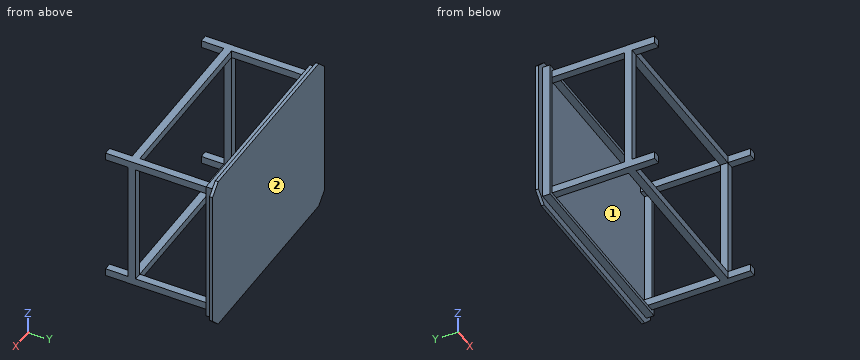
Autodesk Inventor part; units mm, degrees
ref_plane "Plano de trabajo2" through (-617.5, -580, 460) normal (0, 1, 0) x (1, 0, 0)
ref_plane "YZ Plane" through (0, 0, 0) normal (1, 0, 0) x (0, 1, 0)
ref_plane "XZ Plane" through (0, 0, 0) normal (0, 1, 0) x (-1, 0, 0)
sketch "Boceto1" plane through (0, 0, 0) normal (0, 1, 0) x (-1, 0, 0)
  line L0 (692.5, 535) -> (-692.5, 535)
  line L1 (-692.5, 535) -> (-692.5, -535)
  line L2 (-692.5, -535) -> (692.5, -535)
  line L3 (692.5, -535) -> (692.5, 535)
  line L4 (622.5, 535) -> (692.5, 465)
  line L5 (692.5, 0) -> (-692.5, 0)
  line L6 (0, 535) -> (0, -535)
  line L7 (622.5, -535) -> (692.5, -465)
  line L8 (-622.5, 535) -> (-692.5, 465)
  line L9 (-622.5, -535) -> (-692.5, -465)
  arc A0 (-507.7191, -338.4764) -> (-457.7841, -385.927) centre (-457.7841, -335.927) ccw
  line L10 (-457.7841, -385.927) -> (492.0857, -385.927)
  arc A1 (492.0857, -385.927) -> (542.0206, -333.3776) centre (492.0857, -335.927) ccw
  line L11 (542.0206, -333.3776) -> (507.8137, 336.6224)
  arc A2 (507.8137, 336.6224) -> (457.8787, 384.073) centre (457.8787, 334.073) ccw
  line L12 (457.8787, 384.073) -> (-491.991, 384.073)
  arc A3 (-491.991, 384.073) -> (-541.926, 331.5236) centre (-491.991, 334.073) ccw
  line L13 (-541.926, 331.5236) -> (-507.7191, -338.4764)
  point P0 (0, 0)
  point P1 (-692.5, -465)
  point P2 (622.5, -535)
  point P3 (692.5, -465)
  dimension "d0" = 1070
  dimension "d1" = 1385
  dimension "d2" = 692.5
  dimension "d3" = 535
  dimension "d4" = 70
  dimension "d5" = 70
  dimension "d27" = 770
extrude "Extrusión1" add sketch "Boceto1" along normal blind 20 contours L4 L3 L5 L11 A2 L12 L6 L0 | L6 L12 A3 L13 L5 L1 L8 L0 | L3 L7 L2 L6 L10 A1 L11 L5 | L12 A2 L11 L5 L6 | L6 L5 L13 A3 L12 | L11 A1 L10 L6 L5 | L6 L10 A0 L13 L5 | L5 L13 A0 L10 L6 L2 L9 L1
sketch "Boceto2" plane through (0, 0, 0) normal (0, -1, 0) x (1, 0, 0)
  line L0 (-642.5, 485) -> (642.5, 485)
  line L1 (642.5, 485) -> (642.5, -485)
  line L2 (642.5, -485) -> (-642.5, -485)
  line L3 (-642.5, -485) -> (-642.5, 485)
  line L4 (-622.5, 535) -> (622.5, 535)
  line L5 (-692.5, -465) -> (-692.5, 465)
  line L6 (622.5, -535) -> (-622.5, -535)
  line L7 (692.5, 465) -> (692.5, -465)
  line L8 (-617.5, 460) -> (617.5, 460)
  line L9 (617.5, 460) -> (617.5, -460)
  line L10 (617.5, -460) -> (-617.5, -460)
  line L11 (-617.5, -460) -> (-617.5, 460)
  point P0 (0, 0)
  dimension "d8" = 50
  dimension "d9" = 50
  dimension "d10" = 50
  dimension "d11" = 50
  dimension "d12" = 25
  dimension "d13" = 25
  dimension "d14" = 25
  dimension "d15" = 25
extrude "Extrusión2" add sketch "Boceto2" along normal blind 50
sketch "Boceto3" plane through (0, 0, 0) normal (0, -1, 0) x (1, 0, 0)
  line L0 (-617.5, 460) -> (617.5, 460)
  line L1 (-617.5, 460) -> (-567.5, 460)
  line L2 (-567.5, 460) -> (-567.5, 410)
  line L3 (-567.5, 410) -> (-617.5, 410)
  line L4 (-617.5, 410) -> (-617.5, 460)
  line L5 (0, 460) -> (0, -460)
  line L6 (617.5, -460) -> (-617.5, -460)
  line L7 (-617.5, 460) -> (-617.5, -460)
  line L8 (-617.5, 0) -> (472.5, 0)
  line L9 (617.5, 460) -> (567.5, 460)
  line L10 (567.5, 460) -> (567.5, 410)
  line L11 (567.5, 410) -> (617.5, 410)
  line L12 (617.5, 410) -> (617.5, 460)
  line L13 (-617.5, -460) -> (-567.5, -460)
  line L14 (-567.5, -460) -> (-567.5, -410)
  line L15 (-567.5, -410) -> (-617.5, -410)
  line L16 (-617.5, -410) -> (-617.5, -460)
  line L17 (617.5, -460) -> (567.5, -460)
  line L18 (567.5, -460) -> (567.5, -410)
  line L19 (567.5, -410) -> (617.5, -410)
  line L20 (617.5, -410) -> (617.5, -460)
  point P0 (0, 0)
  point P1 (567.5, 460)
  point P2 (567.5, -460)
  point P3 (-617.5, -410)
  point P4 (-567.5, -460)
  dimension "d18" = 50
  dimension "d19" = 50
extrude "Extrusión3" add sketch "Boceto3" along normal blind 730 contours L0 L12 L11 L10 | L18 L19 L20 L6 | L0 L2 L3 L4 | L15 L14 L6 L7
sketch "Boceto4" plane through (-617.5, -50, 460) normal (0, 0, 1) x (1, 0, 0)
  line L0 (0, 0) -> (0, -680)
  line L1 (0, -530) -> (50, -530)
  line L2 (50, 0) -> (50, -680)
  line L3 (50, -680) -> (0, -680)
  point P0 (617.5, 50)
  dimension "d23" = 150
sketch "Boceto5" plane through (567.5, 0, -410) normal (0, 0, 1) x (1, 0, 0)
  line L0 (0, -50) -> (0, -730)
  line L1 (0, -580) -> (50, -580)
  line L2 (50, -50) -> (50, -730)
  line L3 (50, -730) -> (0, -730)
  point P0 (-567.5, 0)
  dimension "d24" = 150
ref_plane "Plano de trabajo2" through (-617.5, -580, 460) normal (0, 1, 0) x (1, 0, 0)
sketch "Boceto6" plane through (-617.5, -580, 460) normal (0, 1, 0) x (1, 0, 0)
  line L0 (0, 0) -> (50, 0)
  line L1 (1235, 50) -> (1185, 50)
  line L2 (50, 0) -> (1185, 0)
  line L3 (1185, 0) -> (1185, 50)
  line L4 (1185, 50) -> (50, 50)
  line L5 (50, 50) -> (50, 0)
  line L6 (1185, 50) -> (1185, 0)
  line L7 (1235, 50) -> (1235, 870)
  line L8 (1185, 50) -> (1235, 50)
  line L9 (1235, 50) -> (1235, 870)
  line L10 (1235, 870) -> (1185, 870)
  line L11 (1185, 870) -> (1185, 50)
  line L12 (1185, 920) -> (1185, 870)
  line L13 (50, 870) -> (50, 920)
  line L14 (1185, 870) -> (50, 870)
  line L15 (50, 870) -> (50, 920)
  line L16 (50, 920) -> (1185, 920)
  line L17 (1185, 920) -> (1185, 870)
  line L18 (0, 870) -> (0, 50)
  line L19 (50, 870) -> (0, 870)
  line L20 (0, 870) -> (0, 50)
  line L21 (0, 50) -> (50, 50)
  line L22 (50, 50) -> (50, 870)
  point P0 (617.5, 460)
  point P1 (50, 50)
  point P2 (50, 50)
  point P3 (50, 870)
  point P4 (50, 870)
  point P5 (0, 870)
extrude "Extrusión4" add sketch "Boceto6" along normal blind 50 contours L1 L11 L10 L7 | L3 L2 L5 L4 | L21 L18 L19 L22 | L14 L13 L16 L12
equation "\"d9\" = d8"
equation "\"d10\" = d8"
equation "\"d11\" = d9"
equation "\"d13\" = d12"
equation "\"d14\" = d12"
equation "\"d15\" = d12"
equation "\"d18\" = d19"
properties part number "Mesa_Centrado"
Part model, mm, in its own coordinate system. Face numbers are marked on the shaded views. Give positions to 0.01 mm unless a question says otherwise; leave off trailing zeros. Order: outer loops, then holes, each group sorted by start corner. A loop starts at its lowest first (then second) coordinate and runs counter-clockwise, first axis right, second up. Notation, with made-up numbers: (22.25, 72) - (73.25, 72) arc R27 cw to (73.25, 103) - close; hole circle Ø1 at (-39, 47.25). An arc over 180 degrees is marked (long way). Use one line per item in the form item = value.
Item 1: Two-plate mould, pull along X, no slides. Class the marked faces 1 and 2: released by +X, released by -X, zero draft, split by the parting line, or undercut.
Solution:
face_1 = undercut
face_2 = zero draft
Item 2: Slice it at C-C on y = -252.5. Give the cut face in (x, z).
Solution:
outline = (-617.5, -460) - (-567.5, -460) - (-567.5, -410) - (-617.5, -410) - close; (-617.5, 410) - (-567.5, 410) - (-567.5, 460) - (-617.5, 460) - close; (567.5, -460) - (617.5, -460) - (617.5, -410) - (567.5, -410) - close; (567.5, 410) - (617.5, 410) - (617.5, 460) - (567.5, 460) - close
Item 3: Probe probe 1 along X at (y, z) = (-36.5, 296.5); probe 2 along Z at (x, y) = (-612.5, -427.5); probe 3 along Z at (x, y) = (281, -39). List the from-to ranges inside material, lowest first. Write a range as from..to.
Solution:
probe_1 = -642.5..-617.5, 617.5..642.5
probe_2 = -460..-410, 410..460
probe_3 = -485..-460, 460..485
Item 4: Slice it at B-B on z = 344.5. Give the cut face in (x, y).
Solution:
outline = (-692.5, 0) - (-642.5, 0) - (-642.5, -50) - (-617.5, -50) - (-617.5, 0) - (617.5, 0) - (617.5, -50) - (642.5, -50) - (642.5, 0) - (692.5, 0) - (692.5, 20) - (-692.5, 20) - close; (-617.5, -580) - (-567.5, -580) - (-567.5, -530) - (-617.5, -530) - close; (567.5, -580) - (617.5, -580) - (617.5, -530) - (567.5, -530) - close
Item 5: Pin check, flat tips, straight feed: pin 1 Ø15 at (x, y) = (602.5, -259) entering from +Z; pin 2 Ø15 at (x, z) = (600.5, -123) entering from -Y; pin 3 Ø15 at (x, y) = (604.5, -247.5) entering from -Z. Stop position of each tip, or through.
Solution:
pin_1 = 460
pin_2 = -580
pin_3 = -460
Item 6: Slice it at A-A on x = -51.5. Give the cut face in (y, z).
Solution:
outline = (-580, -460) - (-530, -460) - (-530, -410) - (-580, -410) - close; (-580, 410) - (-530, 410) - (-530, 460) - (-580, 460) - close; (-50, -485) - (0, -485) - (0, -535) - (20, -535) - (20, 535) - (0, 535) - (0, 485) - (-50, 485) - (-50, 460) - (0, 460) - (0, -460) - (-50, -460) - close
